The listing builds one solid part. Answer for the finished solid, in the listing's coordinates (mm). Face numbers are marked on the shaded views. A direction names the side the tool comes from. Coordinates: 2 decimals unless noted, no trailing zeros. Order: outer loops, then holes, each group sorted by start corner. A loop starts at its lowest first (then second) coordinate and runs counter-clockwise, first axis right, second up. Notation, with made-up numbers: (18, 69.25) - (52, 69.25) arc R7 cw to (52, 79.25) - close; hole circle Ø10 at (-11.5, 60). An arc over 180 degrees is marked (long way). Use one line per item in the form item = value. Start each with the question number.
Item 1: Section B-B, the plane y = 37 is taken. Write down the section's boundary in (x, z).
Item 2: Consider line 1 along Y through (x, z) = (2.5, 2.55); line 2 along Z through (x, y) = (29.5, 14.5); line 3 along Y through (x, z) = (18.5, 2). Determine where each line is inside the solid, lowest interval first. Write a range as [from, to].
Item 3: A tool of negligible diameter and unlimited length cuts with its end or side. For the marked faces 4, 5, 6, 7 and 8, from which of +Z, -Z, +X, -X, +Y, -Y can it reach the whole face along a straight path? Write none if from no direction.
Item 4: Section D-D, the plane y = 20 is taken. Write down the section's boundary in (x, z).
Item 5: Each of these flat-tipped pins is pushed along its axis until it touches: pin 1 Ø6 at (x, y) = (15.5, 20) entering from -Z; pin 2 Ø4 at (x, y) = (4.5, 25) entering from -Z; pin 3 Ø1.5 at (x, y) = (38.5, 37) entering from -Z; pin 4 Ø0.6 at (x, z) = (1.5, 1.5) entering from -Y. Where does it stop, or does it pass through?
Item 6: The mould has two halves that part along X. Classify the marked faces 1, 2 and 3: released by +X, released by -X, zero draft, split by the parting line, or undercut.
Item 7: Section C-C, the plane x = 8 is taken. Write down the section's boundary in (y, z), and give its area (3 significant figures).
Item 8: Section A-A, the plane z = 5.5 is taken. Write down the section's boundary in (x, y).
from build123d import *

# Parameters (mm, degrees)
SKETCH_1_W          = 40
SKETCH_1_H          = 40
EXTRUDE_1_DEPTH     = 10
SKETCH_2_R          = 1.4
CUT_EXTRUDE_1_DEPTH = 58.445626465
SKETCH_3_R          = 13.5
CUT_EXTRUDE_2_DEPTH = 1
SKETCH_4_W          = 28
SKETCH_4_H          = 8.6
CUT_EXTRUDE_3_DEPTH = 5
CUT_EXTRUDE_4_DEPTH = 6.5
CUT_EXTRUDE_START   = -2.1
CUT_EXTRUDE_5_DEPTH = 2.1
FILLET_2_R          = 2
SKETCH_8_R          = 1.5
CUT_EXTRUDE_6_DEPTH = 58.445626465
CUT_EXTRUDE_START_2 = -0.1
CUT_EXTRUDE_7_DEPTH = 0.1


with BuildPart() as part:
    # Эскиз1 → Бобышка-Вытянуть1 (new body)
    with BuildSketch(Plane.XY):
        with Locations((20, 20)):
            Rectangle(SKETCH_1_W, SKETCH_1_H)
    extrude(amount=EXTRUDE_1_DEPTH)

    # Эскиз2 → Вырез-Вытянуть1 (cut, through all)
    with BuildSketch(Plane.XY.offset(10)):
        with Locations((2.5, 37.5)):
            Circle(SKETCH_2_R)
        with Locations((37.5, 37.5)):
            Circle(SKETCH_2_R)
        with Locations((37.5, 2.5)):
            Circle(SKETCH_2_R)
        with Locations((2.5, 2.5)):
            Circle(SKETCH_2_R)
    extrude(amount=-CUT_EXTRUDE_1_DEPTH, mode=Mode.SUBTRACT)

    # Эскиз3 → Вырез-Вытянуть2 (cut)
    with BuildSketch(Plane.XY.offset(10)):
        with Locations((24.2, 20)):
            Circle(SKETCH_3_R)
    extrude(amount=-CUT_EXTRUDE_2_DEPTH, mode=Mode.SUBTRACT)

    # Эскиз4 → Вырез-Вытянуть3 (cut)
    with BuildSketch(Plane.XZ):
        with Locations((20, 5)):
            Rectangle(SKETCH_4_W, SKETCH_4_H)
    extrude(amount=-CUT_EXTRUDE_3_DEPTH, mode=Mode.SUBTRACT)

    # Эскиз5 → Вырез-Вытянуть4 (cut)
    with BuildSketch(Plane.XY.offset(10)):
        with BuildLine():
            Line((2.5, 35), (0, 35))
            Line((0, 35), (0, 40))
            Line((0, 40), (5, 40))
            Line((5, 40), (5, 37.5))
            ThreePointArc((5, 37.5), (4.267766953, 35.732233047), (2.5, 35))
        make_face()
        with BuildLine():
            Line((35, 40), (35, 37.5))
            ThreePointArc((35, 37.5), (35.732233047, 35.732233047), (37.5, 35))
            Line((37.5, 35), (40, 35))
            Line((40, 35), (40, 40))
            Line((40, 40), (35, 40))
        make_face()
        with BuildLine():
            Line((37.5, 5), (40, 5))
            Line((40, 5), (40, 0))
            Line((40, 0), (35, 0))
            Line((35, 0), (35, 2.5))
            ThreePointArc((35, 2.5), (35.732233047, 4.267766953), (37.5, 5))
        make_face()
        with BuildLine():
            Line((5, 0), (5, 2.5))
            ThreePointArc((5, 2.5), (4.267766953, 4.267766953), (2.5, 5))
            Line((2.5, 5), (0, 5))
            Line((0, 5), (0, 0))
            Line((0, 0), (5, 0))
        make_face()
    extrude(amount=-CUT_EXTRUDE_4_DEPTH, mode=Mode.SUBTRACT)

    # Эскиз6 → Вырез-Вытянуть5 (cut)
    with BuildSketch(Plane(origin=(0, 0, 0), x_dir=(-1, 0, 0), z_dir=(0, 0, -1)).offset(CUT_EXTRUDE_START)):
        with BuildLine():
            Line((-2.5, 35), (0, 35))
            Line((0, 35), (0, 40))
            Line((0, 40), (-5, 40))
            Line((-5, 40), (-5, 37.5))
            ThreePointArc((-5, 37.5), (-4.267766953, 35.732233047), (-2.5, 35))
        make_face()
        with BuildLine():
            Line((-35, 37.5), (-35, 40))
            Line((-35, 40), (-40, 40))
            Line((-40, 40), (-40, 35))
            Line((-40, 35), (-37.5, 35))
            ThreePointArc((-37.5, 35), (-35.732233047, 35.732233047), (-35, 37.5))
        make_face()
        with BuildLine():
            Line((-5, 0), (0, 0))
            Line((0, 0), (0, 5))
            Line((0, 5), (-2.5, 5))
            ThreePointArc((-2.5, 5), (-4.267766953, 4.267766953), (-5, 2.5))
            Line((-5, 2.5), (-5, 0))
        make_face()
        with BuildLine():
            Line((-40, 5), (-40, 0))
            Line((-40, 0), (-35, 0))
            Line((-35, 0), (-35, 2.5))
            ThreePointArc((-35, 2.5), (-35.732233047, 4.267766953), (-37.5, 5))
            Line((-37.5, 5), (-40, 5))
        make_face()
    extrude(amount=CUT_EXTRUDE_5_DEPTH, mode=Mode.SUBTRACT)

    # Скругление2
    fillet_2_edges = [part.edges().sort_by_distance(p)[0] for p in [
        (0, 40, 2.8),
        (40, 40, 2.8),
        (40, 0, 2.8),
        (0, 0, 2.8),
    ]]
    fillet(fillet_2_edges, radius=FILLET_2_R)

    # Эскиз8 → Вырез-Вытянуть6 (cut, through all)
    with BuildSketch(Plane.XY.offset(10)):
        with Locations((40, 12)):
            Circle(SKETCH_8_R)
    extrude(amount=-CUT_EXTRUDE_6_DEPTH, mode=Mode.SUBTRACT)

    # Эскиз9 → Вырез-Вытянуть7 (cut)
    with BuildSketch(Plane(origin=(0, 0, 0), x_dir=(-1, 0, 0), z_dir=(0, 0, -1)).offset(CUT_EXTRUDE_START_2)):
        with BuildLine():
            Line((-40, 13.5), (-33.314476962, 15.672794987))
            ThreePointArc((-33.314476962, 15.672794987), (-7.214062681, 25.702614039), (-32.115767056, 12.985145144))
            Line((-32.115767056, 12.985145144), (-39.536370891, 10.573448897))
            ThreePointArc((-39.536370891, 10.573448897), (-38.518476012, 12.234705502), (-40, 13.5))
        make_face()
    extrude(amount=CUT_EXTRUDE_7_DEPTH, mode=Mode.SUBTRACT)


solid = part.part
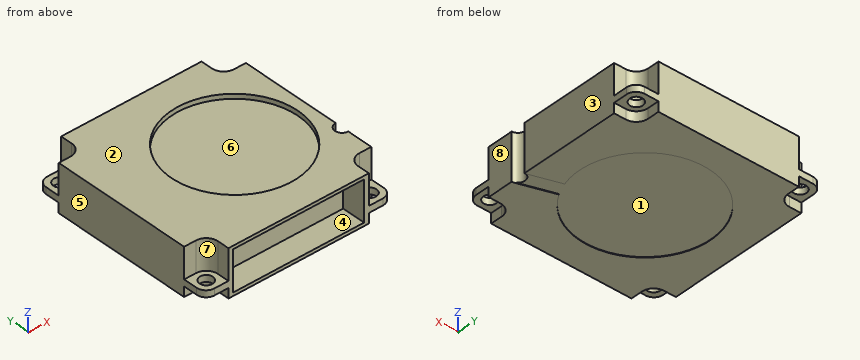
Response:
q1.outline = (0, 2.1) - (1.19, 2.1) - (1.19, 3.5) - (0, 3.5) - close; (3.81, 2.1) - (4.95, 2.1) - (4.95, 0) - (35.05, 0) - (35.05, 2.1) - (36.19, 2.1) - (36.19, 3.5) - (35.05, 3.5) - (35.05, 10) - (4.95, 10) - (4.95, 3.5) - (3.81, 3.5) - close; (38.81, 2.1) - (40, 2.1) - (40, 3.5) - (38.81, 3.5) - close
q2.line_1 = [0, 1.1], [3.9, 36.1], [38.9, 40]
q2.line_2 = [0.1, 9]
q2.line_3 = [5, 40]
q3.face_4 = -Y
q3.face_5 = +Z, -Z, -X, +Y, -Y
q3.face_6 = +Z
q3.face_7 = +Z, -X, -Y
q3.face_8 = +Z, -Z, +X, +Y, -Y
q4.outline = (0, 0) - (6, 0) - (6, 0.1) - (34, 0.1) - (34, 0) - (40, 0) - (40, 10) - (37.7, 10) - (37.7, 9) - (10.7, 9) - (10.7, 10) - (0, 10) - close
q5.pin_1 = 0.1
q5.pin_2 = 0
q5.pin_3 = 2.1
q5.pin_4 = 5
q6.face_1 = undercut
q6.face_2 = zero draft
q6.face_3 = released by +X
q7.outline = (0, 0) - (12.79, 0) - (12.79, 0.1) - (27.21, 0.1) - (27.21, 0) - (40, 0) - (40, 10) - (0, 10) - (0, 9.3) - (5, 9.3) - (5, 0.7) - (0, 0.7) - close
q7.area = 356 mm2
q8.outline = (0, 5) - (2.5, 5) arc R2.5 cw to (5, 2.5) - (5, 0) - (6, 0) - (6, 5) - (34, 5) - (34, 0) - (35, 0) - (35, 2.5) arc R2.5 cw to (37.5, 5) - (40, 5) - (40, 10.5) arc R1.5 cw to (40, 13.5) - (40, 35) - (37.5, 35) arc R2.5 cw to (35, 37.5) - (35, 40) - (5, 40) - (5, 37.5) arc R2.5 cw to (2.5, 35) - (0, 35) - close
